Part model, mm, in its own coordinate system. A direction names the side the tool comes from. Give positions to 0.01 mm unless a question says otherwise; leave off trailing zeros. Write each loop counter-clockwise with the first axis right and the second up, starting at its lowest first coordinate (ties: lowest second). Pieces come first, ordered by that corner, then holes.
from build123d import *

# Parameters (mm, degrees)
SKETCH_1_R          = 3.25
SKETCH_1_R_2        = 1.7
EXTRUDE_1_DEPTH     = 5
CUT_EXTRUDE_START   = 5
SKETCH_1_4_R        = 3.25
CUT_EXTRUDE_1_DEPTH = 1.5
CUT_EXTRUDE_START_2 = -5
SKETCH_1_5_R        = 3.25
CUT_EXTRUDE_2_DEPTH = 1.5
CUT_EXTRUDE_START_3 = 2.43999
SKETCH_2_R          = 3
CUT_EXTRUDE_3_DEPTH = 3.5


with BuildPart() as part:
    # Эскиз1 → Бобышка-Вытянуть1 (new, symmetric)
    # profile 1 of 4: a face of its own
    with BuildSketch(Plane.XY):
        with BuildLine():
            Line((-0.402987496, 15.3), (-6, 15.3))
            ThreePointArc((-6, 15.3), (-6.353553391, 15.153553391), (-6.5, 14.8))
            Line((-6.5, 14.8), (-6.5, 12.650103769))
            ThreePointArc((-6.5, 12.650103769), (-6.409576022, 12.363315551), (-6.171010072, 12.180257459))
            Line((-6.171010072, 12.180257459), (-4.136019248, 11.439581372))
            ThreePointArc((-4.136019248, 11.439581372), (-3.91562246, 11.280863122), (-3.810716101, 11.0303419))
            ThreePointArc((-3.810716101, 11.0303419), (-3.681235408, 6.344733002), (-4.428694025, 1.717314542))
            ThreePointArc((-4.428694025, 1.717314542), (-1.542362614, 4.492618119), (2.439992619, 4.07540624))
            Line((2.439992619, 4.07540624), (0.085601919, 14.90620915))
            ThreePointArc((0.085601919, 14.90620915), (-0.089223711, 15.189297171), (-0.402987496, 15.3))
        make_face()
    # profile 2 of 4: a face of its own
    with BuildSketch(Plane.XY):
        with BuildLine():
            ThreePointArc((4.75, 0), (4.13233983, 2.342278278), (2.439992619, 4.07540624))
            ThreePointArc((2.439992619, 4.07540624), (-1.542362614, 4.492618119), (-4.428694025, 1.717314542))
            ThreePointArc((-4.428694025, 1.717314542), (-4.75, 0), (-4.428694025, -1.717314542))
            ThreePointArc((-4.428694025, -1.717314542), (-4.378812236, -1.835465051), (-4.329537208, -1.953869895))
            ThreePointArc((-4.329537208, -1.953869895), (-1.385071911, -4.543575222), (2.503326388, -4.036812727))
            ThreePointArc((2.503326388, -4.036812727), (4.150499991, -2.309945849), (4.75, 0))
        make_face()
        Circle(SKETCH_1_R, mode=Mode.SUBTRACT)
    # profile 3 of 4: a face of its own
    with BuildSketch(Plane.XY):
        Circle(SKETCH_1_R)
        Circle(SKETCH_1_R_2, mode=Mode.SUBTRACT)
    # profile 4 of 4: a face of its own
    with BuildSketch(Plane.XY):
        with BuildLine():
            Line((0.359159672, -14.7), (2.503326388, -4.036812727))
            ThreePointArc((2.503326388, -4.036812727), (-1.385071911, -4.543575222), (-4.329537208, -1.953869895))
            ThreePointArc((-4.329537208, -1.953869895), (-2.65175784, -8.216516162), (-2.640840328, -14.7))
            Line((-2.640840328, -14.7), (-2.640840328, -22.7))
            ThreePointArc((-2.640840328, -22.7), (-2.494393719, -23.053553391), (-2.140840328, -23.2))
            Line((-2.140840328, -23.2), (1.359159672, -23.2))
            Line((1.359159672, -23.2), (3.505606281, -21.053553391))
            ThreePointArc((3.505606281, -21.053553391), (3.613992657, -20.508658284), (3.152052891, -20.2))
            Line((3.152052891, -20.2), (0.859159672, -20.2))
            ThreePointArc((0.859159672, -20.2), (0.505606281, -20.053553391), (0.359159672, -19.7))
            Line((0.359159672, -19.7), (0.359159672, -14.7))
        make_face()
    extrude(amount=EXTRUDE_1_DEPTH, both=True)

    # Эскиз1<4> → Вырез-Вытянуть1 (cut)
    with BuildSketch(Plane.XY.offset(CUT_EXTRUDE_START)):
        Circle(SKETCH_1_4_R)
    extrude(amount=-CUT_EXTRUDE_1_DEPTH, mode=Mode.SUBTRACT)

    # Эскиз1<5> → Вырез-Вытянуть2 (cut)
    with BuildSketch(Plane.XY.offset(CUT_EXTRUDE_START_2)):
        Circle(SKETCH_1_5_R)
    extrude(amount=CUT_EXTRUDE_2_DEPTH, mode=Mode.SUBTRACT)

    # Эскиз2 → Вырез-Вытянуть3 (cut)
    with BuildSketch(Plane(origin=(0, 0.681903291, 0), x_dir=(0, 0, -1), z_dir=(1, 0, 0)).offset(CUT_EXTRUDE_START_3)):
        with Locations((0, 9.818096709)):
            Circle(SKETCH_2_R)
    extrude(amount=-CUT_EXTRUDE_3_DEPTH, mode=Mode.SUBTRACT)


solid = part.part
1) Saw through at B-B (y = 0). Write the cut outline in (x, z).
Check result:
outline: (-4.75, -5) - (-3.25, -5) - (-3.25, -3.5) - (-1.7, -3.5) - (-1.7, 3.5) - (-3.25, 3.5) - (-3.25, 5) - (-4.75, 5) - close; (1.7, -3.5) - (3.25, -3.5) - (3.25, -5) - (4.75, -5) - (4.75, 5) - (3.25, 5) - (3.25, 3.5) - (1.7, 3.5) - close
2) Saw through at A-A (z = 4.25). Write the cut outline in (x, y), and give its area (3 significant figures).
Check result:
outline: (-6.5, 12.65) arc R0.5 ccw to (-6.17, 12.18) - (-4.14, 11.44) arc R0.5 cw to (-3.81, 11.03) arc R25 cw to (-4.43, 1.72) arc R4.75 ccw to (-4.43, -1.72) arc R25 cw to (-4.33, -1.95) arc R25 cw to (-2.64, -14.7) - (-2.64, -22.7) arc R0.5 ccw to (-2.14, -23.2) - (1.36, -23.2) - (3.51, -21.05) arc R0.5 ccw to (3.15, -20.2) - (0.86, -20.2) arc R0.5 cw to (0.36, -19.7) - (0.36, -14.7) - (2.5, -4.04) arc R4.75 ccw to (2.44, 4.08) - (0.09, 14.91) arc R0.5 ccw to (-0.4, 15.3) - (-6, 15.3) arc R0.5 ccw to (-6.5, 14.8) - close; hole circle Ø6.5 at (0, 0)
area: 177 mm2
3) Mould opens along X. For faces 4 (the cylindrical face through (-2.579, -1.978, -4.26)), 5 (the flat face through (0.359, -17, 0)), 6 (the flat face through (0, -23.2, 0)) say: +X half, -X half, draft (parallel to the pull), parting line (faces both ways), or undercut.
Check result:
face 4: undercut
face 5: +X half
face 6: draft
4) Flat gauge pins, fed straight in: P1, Ø0.7, axis at x = 1.5, z = -0.5, coming from the +Y side; P2, Ø3, axis at x = 0, y = 0, coming from the +Z side; P3, Ø1.5, axis at y = -18, z = 0.5, coming from the +X side; P4, Ø5, axis at x = 0, y = 0, coming from the -Z side. Where does each tip first touch, or does it go through?
Check result:
P1: stops at y = 7.62
P2: passes through
P3: stops at x = 0.36
P4: stops at z = -3.5
5) Saw through at D-D (y = 10.5). Write the cut outline in (x, z).
Check result:
outline: (-3.75, -5) - (1.04, -5) - (1.04, -3) - (-1.06, -3) - (-1.06, 3) - (1.04, 3) - (1.04, 5) - (-3.75, 5) - close
6) Drill centre lines: L1, parallel to X at y = 0, z = -2.5; L2, parallel to X at y = -17.5, z = 3.5; L3, parallel to Y at x = 0, z = -4. Where is each one in solid material? Low to high.
Check result:
L1: x = -4.75 to -1.7, 1.7 to 4.75
L2: x = -2.64 to 0.36
L3: y = -23.2 to -3.25, 3.25 to 15.1
7) 3-axis set-ups, long thin cutter, end or side, ignore diameter. For faces 1 (the flat face through (-1.06, 11, 0)), 2 (the flat face through (-5.168, 11.815, 0.07)), 3 (the flat face through (1.416, -9.443, 0.07)): which of +Z, -Z, +X, -X, +Y, -Y reach the whole face in a straight line?
Check result:
face 1: +X
face 2: +Z, -Z, -X
face 3: +Z, -Z, +X
8) Saw through at C-C (z = 1.75). Write the cut outline in (x, y).
Check result:
outline: (-6.5, 12.65) arc R0.5 ccw to (-6.17, 12.18) - (-4.14, 11.44) arc R0.5 cw to (-3.81, 11.03) arc R25 cw to (-4.43, 1.72) arc R4.75 ccw to (-4.43, -1.72) arc R25 cw to (-4.33, -1.95) arc R25 cw to (-2.64, -14.7) - (-2.64, -22.7) arc R0.5 ccw to (-2.14, -23.2) - (1.36, -23.2) - (3.51, -21.05) arc R0.5 ccw to (3.15, -20.2) - (0.86, -20.2) arc R0.5 cw to (0.36, -19.7) - (0.36, -14.7) - (2.5, -4.04) arc R4.75 ccw to (2.44, 4.08) - (1.57, 8.06) - (-1.06, 8.06) - (-1.06, 12.94) - (0.51, 12.94) - (0.09, 14.91) arc R0.5 ccw to (-0.4, 15.3) - (-6, 15.3) arc R0.5 ccw to (-6.5, 14.8) - close; hole circle Ø3.4 at (0, 0)
